Build history of the part. All positions in model axes, mm. A direction names the side the tool comes from. Round coordinates to 2 decimals unless told otherwise and drop trailing zeros. Order: outer loops, then holes, each group sorted by start corner. A loop starts at its lowest first (then second) coordinate and runs counter-clockwise, first axis right, second up. Notation, with made-up numbers: M -40,35.5 L 17,35.5 A29 cw 17,68.5 Z; hole C -25.75,67 d10. An arc over 180 degrees is marked long. One line per question, with ' | ' between items. Start each with the question number.
from build123d import *

# Parameters (mm, degrees)
F_2_7_2_7_DIAMETER_HOLE1_REACH  = 24.913
F_2_7_2_7_DIAMETER_HOLE1_BORE_R = 1.35


with BuildPart() as part:
    # Sketch1 → Revolve1 (revolve)
    with BuildSketch(Plane(origin=(0, 0, 0), x_dir=(0, 0, -1), z_dir=(1, 0, 0)), mode=Mode.PRIVATE) as revolve1_sk:
        Polygon((-4.1, 0), (-5, 0), (-6, 1), (-10, 1), (-10, 5), (-4.1, 5), align=None)
    revolve(revolve1_sk.sketch.rotate(Axis((0, 0, 0), (0, 1, 0)), 180), axis=Axis((0, 0, 0), (0, 1, 0)))

    # Ø2.7 (2.7) Diameter Hole1 bore → Ø2.7 (2.7) Diameter Hole1 (cut, up to next)
    with BuildSketch(Plane(origin=(0, 0, -10), x_dir=(-1, 0, 0), z_dir=(0, 0, -1)), mode=Mode.PRIVATE) as f_2_7_2_7_diameter_hole1_sk1:
        with Locations((0, 3)):
            Circle(F_2_7_2_7_DIAMETER_HOLE1_BORE_R)
    f_2_7_2_7_diameter_hole1_tool1 = extrude(f_2_7_2_7_diameter_hole1_sk1.sketch, amount=-F_2_7_2_7_DIAMETER_HOLE1_REACH, mode=Mode.PRIVATE) & part.part
    add(f_2_7_2_7_diameter_hole1_tool1.solids().sort_by_distance((0, 3, -10))[0], mode=Mode.SUBTRACT)


solid = part.part
Item 1: Flat gauge pins, fed straight in: pin 1 (1.5 mm diameter, centred on x = -5, y = 3, fed in from -Z); pin 2 (1 mm diameter, centred on y = 4, z = 4.5, fed in from +X); pin 3 (1 mm diameter, centred on y = 2.5, z = 4, fed in from -X). Where does each tip first touch, or does it go through?
Item 2: Wall check: line 1 along X through (y, z) = (3.6, 0); line 2 along X through (y, z) = (3, -8); line 3 along Z through (x, y) = (1.5, 3). Give the ranges that are in metal, low to high. Write a range as [from, to].
Item 3: Cut at B-B on z = 0. Write the cut outline in (x, y).
Item 4: Cut at A-A on x = 0. Write the cut outline in (y, z), then the cut area to 3 significant figures.
Item 5: Tool access for faces 4 (the face through (0.29, 1.68, -6.98)), 5 (the face through (-2, 0, -4)): list every direction of +Z, -Z, +X, -X, +Y, -Y with a clear straight run to the whole face (end or side of a thin tool).
Item 6: Two-plate mould, pull along X, no slides. Class faces 1 (the face through (-0.18, 2.465, 4.096)), 2 (the face through (7, 1, 0)), 3 (the face through (0, 3, 10)): +X half, -X half, draft (parallel to the pull), parting line (faces both ways), or undercut.
Item 7: Cut at C-C on y = 0.5. Write the cut outline in (x, z).
Item 8: Cut at D-D on z = 8. Write the cut outline in (x, y), then the cut area to 3 significant figures.
Results found:
1) pin 1: stops at z = -9.05 | pin 2: stops at x = 9.17 | pin 3: stops at x = -9.37
2) line 1: x = [-10, -4.1], [4.1, 10] | line 2: x = [-6, -1.35], [1.35, 6] | line 3: z = [-9.89, -3.82], [3.82, 9.89]
3) outline: M -10,1 L -6,1 L -5,0 L -4.1,0 L -4.1,5 L -10,5 Z; M 4.1,0 L 5,0 L 6,1 L 10,1 L 10,5 L 4.1,5 Z
4) outline: M 0,-5 L 1,-6 L 1,-10 L 1.65,-10 L 1.65,-4.1 L 0,-4.1 Z; M 0,4.1 L 5,4.1 L 5,10 L 1,10 L 1,6 L 0,5 Z; M 4.35,-10 L 5,-10 L 5,-4.1 L 4.35,-4.1 Z | area: 34.1 mm^2
5) face 4: -Z | face 5: +Z, -Z, +X, -X, -Y
6) face 1: undercut | face 2: draft | face 3: parting line
7) outline: C 0,0 d11; hole C 0,0 d8.2
8) outline: M -6,1 L 6,1 L 6,5 L -6,5 Z | area: 48.0 mm^2
